from build123d import *

# Parameters (mm, degrees)
SKETCH1_W           = 19.106827842
SKETCH1_H           = 12
SKETCH1_R           = 1.5
SKETCH1_R_2         = 1.6
SKETCH1_R_3         = 1.65
SKETCH1_R_4         = 1.55
BOSS_EXTRUDE1_DEPTH = 2.25


with BuildPart() as part:
    # Sketch1 → Boss-Extrude1 (new body)
    with BuildSketch(Plane(origin=(0, 0, 0), x_dir=(1, 0, 0), z_dir=(0, 1, 0))):
        Rectangle(SKETCH1_W, SKETCH1_H)
        with Locations((-6.925755231, 1.836983108)):
            Circle(SKETCH1_R, mode=Mode.SUBTRACT)
        with Locations((7.098878727, 1.797303867)):
            Circle(SKETCH1_R_2, mode=Mode.SUBTRACT)
        with Locations((7.098878727, -2.077930101)):
            Circle(SKETCH1_R_3, mode=Mode.SUBTRACT)
        with Locations((-6.925755231, -2.077930101)):
            Circle(SKETCH1_R_4, mode=Mode.SUBTRACT)
        Polygon((2.685, 1.550185473), (0, 3.100370946), (-2.685, 1.550185473), (-2.685, -1.550185473), (0, -3.100370946), (2.685, -1.550185473), align=None, mode=Mode.SUBTRACT)
    extrude(amount=BOSS_EXTRUDE1_DEPTH)


solid = part.part
Could you check a few things on this model? Use its own coordinates, in mm. A direction names the side the tool comes from. Round coordinates to 2 decimals unless told otherwise and drop trailing zeros. Order: outer loops, then holes, each group sorted by start corner. A loop starts at its lowest first (then second) coordinate and runs counter-clockwise, first axis right, second up.
(1) Imagine slicing it at B-B (z = 2.5). Write out the boundary of the cut face in (x, y).
Response values:
outline: (-9.55, 0) - (-8.42, 0) - (-8.42, 2.25) - (-9.55, 2.25) - close; (-5.43, 0) - (-1.04, 0) - (-1.04, 2.25) - (-5.43, 2.25) - close; (1.04, 0) - (5.5, 0) - (5.5, 2.25) - (1.04, 2.25) - close; (8.69, 0) - (9.55, 0) - (9.55, 2.25) - (8.69, 2.25) - close
(2) Imagine slicing it at D-D (x = 2.5). Write out the boundary of the cut face in (y, z), plus the area to 3 significant figures.
Response values:
outline: (0, -6) - (2.25, -6) - (2.25, -1.66) - (0, -1.66) - close; (0, 1.66) - (2.25, 1.66) - (2.25, 6) - (0, 6) - close
area: 19.5 mm2
(3) Imagine slicing it at C-C (x = 7.25). Write out the boundary of the cut face in (y, z), plus the area to 3 significant figures.
Response values:
outline: (0, -6) - (2.25, -6) - (2.25, -3.39) - (0, -3.39) - close; (0, -0.2) - (2.25, -0.2) - (2.25, 0.43) - (0, 0.43) - close; (0, 3.72) - (2.25, 3.72) - (2.25, 6) - (0, 6) - close
area: 12.4 mm2
(4) If we mould it in two halves opening along X, with no side actions, what happens to faces 3 (the cylindrical face through (-8.03, 1.11, -2.85)), 4 (the cylindrical face through (8.625, 1.109, -2.278)), 5 (the flat face through (-9.553, 1, 0)), 6 (the flat face through (0, 1, -6))? For each: released by +X, released by -X, zero draft, split by the parting line, or undercut.
Response values:
face 3: undercut
face 4: undercut
face 5: released by -X
face 6: zero draft
(5) Imagine slicing it at A-A (z = 0). Write out the boundary of the cut face in (x, y) (3 decimals).
Response values:
outline: (-9.553, 0) - (-2.685, 0) - (-2.685, 2.25) - (-9.553, 2.25) - close; (2.685, 0) - (9.553, 0) - (9.553, 2.25) - (2.685, 2.25) - close
(6) Please list where these lines run through material, in increasing order: line 1 along Z through (x, y) = (8.5, 0.9); line 2 along Z through (x, y) = (-6.5, 1.1); line 3 along X through (y, z) = (0.95, 3.5).
Response values:
line 1: z = -6 to -2.57, -1.02 to 1.21, 2.95 to 6
line 2: z = -6 to -3.28, -0.4 to 0.59, 3.57 to 6
line 3: x = -9.55 to -7.54, -6.31 to 6.26, 7.94 to 9.55
(7) Which directions (+Z, -Z, +X, -X, +Y, -Y) give clear straight access to the entire face, cutting with the end or side of a thin tool? Please do faces 1 (the flat face through (-2, 0, 3)), 2 (the flat face through (1.32, 1.11, 2.34)).
Response values:
face 1: +Z, -Z, +X, -X, -Y
face 2: +Y, -Y
(8) I'm going to push a flat-ended pin straight in: pin 1 (2 mm diameter, centred on x = 4, z = 2.5, fed in from -Y). Where does the tip first touch, or does it pass through?
Response values:
pin 1: stops at y = 0
